```python
from build123d import *

# Parameters (mm, degrees)
EXTRUDE_1_DEPTH     = 6
CUT_EXTRUDE_1_DEPTH = 10


with BuildPart() as part:
    # Эскиз2 → Бобышка-Вытянуть1 (new body)
    with BuildSketch(Plane.XY):
        Polygon((0, 0), (-9, 0), (-9, 5.45), (0, 5.45), (0, 15.45), (5.45, 15.45), (5.45, 45.45), (0, 45.45), (0, 55.45), (-9, 55.45), (-9, 60.9), (-39.35, 60.9), (-39.35, 55.45), (-198.65, 55.45), (-198.65, 60.9), (-229, 60.9), (-229, 55.45), (-238, 55.45), (-238, 45.45), (-243.45, 45.45), (-243.45, 15.45), (-238, 15.45), (-238, 5.45), (-229, 5.45), (-229, 0), (-238, 0), (-238, -84.65), (-244, -84.65), (-244, -115), (-238, -115), (-238, -144.65), (-244, -144.65), (-244, -175), (-238, -175), (-238, -204.65), (-244, -204.65), (-244, -235), (-238, -235), (-238, -250), (-229, -250), (-229, -256), (-199, -256), (-199, -250), (-39, -250), (-39, -256), (-9, -256), (-9, -250), (0, -250), (0, -235), (6, -235), (6, -204.65), (0, -204.65), (0, -175), (6, -175), (6, -144.65), (0, -144.65), (0, -115), (6, -115), (6, -84.65), (0, -84.65), align=None)
        Polygon((-199, 0), (-199, 5.45), (-139, 5.45), (-139, 10.9), (-99, 10.9), (-99, 5.45), (-39, 5.45), (-39, 0), align=None, mode=Mode.SUBTRACT)
    extrude(amount=EXTRUDE_1_DEPTH)

    # Эскиз4 → Вырез-Вытянуть1 (cut)
    with BuildSketch(Plane.XY.offset(6)):
        Polygon((-114, -100), (-113, -100), (-113, -110), (-125, -110), (-125, -100), (-124, -100), (-124, 0), (-114, 0), align=None)
    extrude(amount=-CUT_EXTRUDE_1_DEPTH, mode=Mode.SUBTRACT)


solid = part.part
```
Source: CAD feature listing. Evaluate the final solid. Frame: model axes, mm. Give positions to 0.01 mm unless a question says otherwise; leave off trailing zeros. Loops run counter-clockwise (first coordinate to the right, second up) from the corner with the lowest first, then second, coordinate; pieces in that order, holes last. Notation, with made-up numbers: M 64,-4 L 121,-4 A19 cw 121,33 Z; hole C 68.5,21 d3. An arc over 180 degrees is marked long. Put each result on its own line as item: value.
Q1. Section C-C (y = -197.5). Return the cut outline in (x, z), and give its area (3 significant figures).
Response values:
outline: M -238,0 L 0,0 L 0,6 L -238,6 Z
area: 1,430 mm²
Q2. Line query: probe 1 along X at (y, z) = (-96, 3.25); probe 2 along Y at (x, z) = (-105.5, 1); probe 3 along Y at (x, z) = (-79, 5.35). Output: solid intervals per line, ascending. Write a range as [from, to].
Response values:
probe 1: x = [-244, -124], [-114, 6]
probe 2: y = [-250, 0], [10.9, 55.45]
probe 3: y = [-250, 0], [5.45, 55.45]
Q3. Section A-A (y = -62). Return the cut outline in (x, z).
Response values:
outline: M -238,0 L -124,0 L -124,6 L -238,6 Z; M -114,0 L 0,0 L 0,6 L -114,6 Z
Q4. Section B-B (x = -83). Return the cut outline in (y, z).
Response values:
outline: M -250,0 L 0,0 L 0,6 L -250,6 Z; M 5.45,0 L 55.45,0 L 55.45,6 L 5.45,6 Z
Q5. Pin query (flat end, axial travel): P1, Ø1.8, axis at x = -6.5, z = 1.5, coming from the -Y side; P2, Ø1, axis at y = -24.5, z = 2, coming from the -X side; P3, Ø3, axis at x = -242, z = 3, coming from the +Y side; P4, Ø1, axis at x = -43.5, y = -29, coming from the -Z side. Return the tip coordinate at first contact, or that it passes through.
Response values:
P1: stops at y = -250
P2: stops at x = -238
P3: stops at y = 45.45
P4: stops at z = 0
